Design review of the part shown in the three views and the two pictorial views. Dimensions are in mm from the part's minimum x, y and z. Give positions to 0.01 mm unless a question says otherwise; leave off trailing zeros. Loops run counter-clockwise (first coordinate to the right, second up) from the corner with the lowest first, then second, coordinate; pieces in that order, holes last. Notation, with made-up numbers: (-39, 89) -> (-5, 89) arc R32 ccw to (-5, 123) -> close; hole circle Ø3 at (77, -33.5). An arc over 180 degrees is marked (long way). Use CSV: the item, a comma, the result in double quotes. Start each with the question number.
Item 1: Wall thickness on line 1 along Y through (x, z) = (70, 5.9); line 2 along X through (y, z) = (54, 1); line 3 along Y through (x, z) = (37.5, 5.55): over which ranges is each line inside the solid? List them lowest first. Write a range as from..to.
Item 2: Clearance check with flat-ended pins moving along their axes: pin 1 (3 mm diameter, centred on x = 66, y = 42.5, fed in from -Z); pin 2 (4 mm diameter, centred on y = 34, z = 2.5, fed in from -X); pin 3 (0.5 mm diameter, centred on y = 28.5, z = 0.5, fed in from -X); pin 4 (1.5 mm diameter, centred on x = 9, z = 1.5, fed in from -Y). State where each tip first meets the part, or that it passes through.
Item 3: We need section D-D (z = 6). State the section outline as (x, y) points.
Item 4: We need section A-A (y = 5). State the section outline as (x, z) points, plus the area to 3 significant figures.
Item 5: We need section B-B (x = 37.5). State the section outline as (y, z) points.
Item 6: The part is to be moulded in two halves that separate along X. For the marked faces 1, 2 and 3, say which applies: +X half, -X half, draft (parallel to the pull), parting line (faces both ways), or undercut.
Item 7: We need section C-C (y = 37.5). State the section outline as (x, z) points.
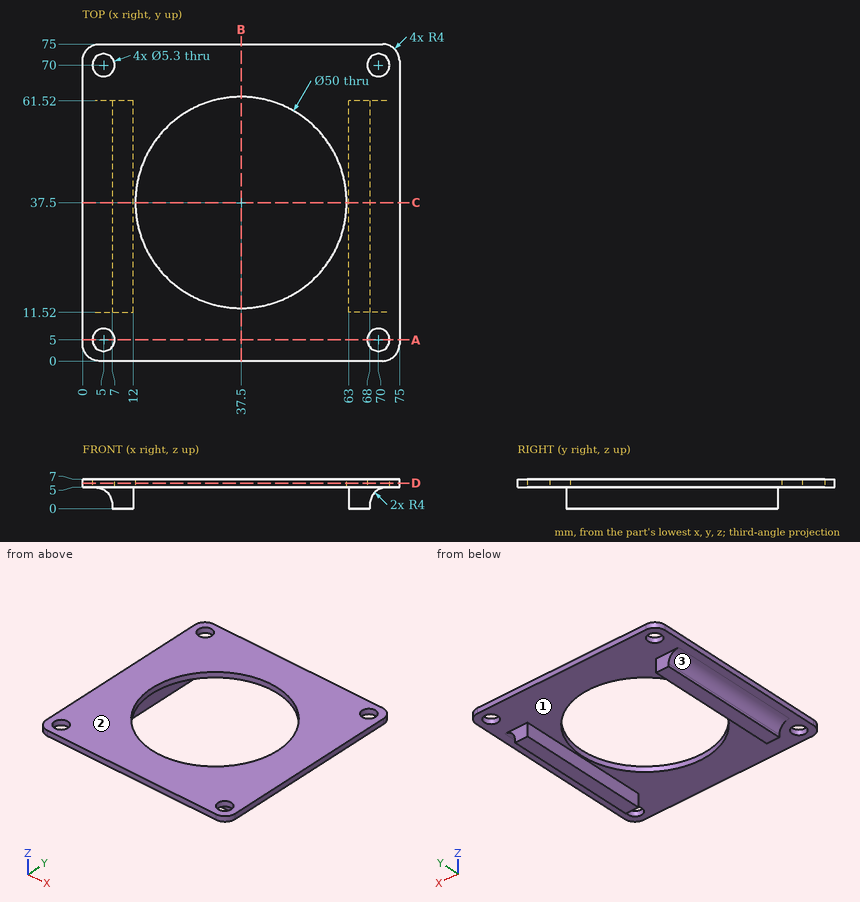
Results found:
1,line 1,"0..2.35, 7.65..67.35, 72.65..75"
1,line 2,"7..12, 63..68"
1,line 3,"0..12.5, 62.5..75"
2,pin 1,"z = 0"
2,pin 2,"x = 4.94"
2,pin 3,"x = 7"
2,pin 4,"y = 11.52"
3,outline,"(0, 4) arc R4 ccw to (4, 0) -> (71, 0) arc R4 ccw to (75, 4) -> (75, 71) arc R4 ccw to (71, 75) -> (4, 75) arc R4 ccw to (0, 71) -> close; hole circle Ø5.3 at (5, 5); hole circle Ø5.3 at (5, 70); hole circle Ø50 at (37.5, 37.5); hole circle Ø5.3 at (70, 5); hole circle Ø5.3 at (70, 70)"
4,outline,"(0, 5) -> (2.35, 5) -> (2.35, 7) -> (0, 7) -> close; (7.65, 5) -> (67.35, 5) -> (67.35, 7) -> (7.65, 7) -> close; (72.65, 5) -> (75, 5) -> (75, 7) -> (72.65, 7) -> close"
4,area,"129 mm²"
5,outline,"(0, 5) -> (12.5, 5) -> (12.5, 7) -> (0, 7) -> close; (62.5, 5) -> (75, 5) -> (75, 7) -> (62.5, 7) -> close"
6,face 1,"undercut"
6,face 2,"draft"
6,face 3,"-X half"
7,outline,"(0, 5) -> (3, 5) arc R4 cw to (7, 1) -> (7, 0) -> (12, 0) -> (12, 5) -> (12.5, 5) -> (12.5, 7) -> (0, 7) -> close; (62.5, 5) -> (63, 5) -> (63, 0) -> (68, 0) -> (68, 1) arc R4 cw to (72, 5) -> (75, 5) -> (75, 7) -> (62.5, 7) -> close"
